Autodesk Inventor part; units mm, degrees
ref_plane "YZ Plane" through (0, 0, 0) normal (1, 0, 0) x (0, 1, 0)
ref_plane "XZ Plane" through (0, 0, 0) normal (0, 1, 0) x (-1, 0, 0)
ref_plane "XY Plane" through (0, 0, 0) normal (0, 0, 1) x (1, 0, 0)
sketch "スケッチ1" plane through (0, 0, 0) normal (0, 0, 1) x (1, 0, 0)
  line L0 (-23, 23) -> (23, 23)
  line L1 (23, 23) -> (23, -23)
  line L2 (23, -23) -> (-23, -23)
  line L3 (-23, -23) -> (-23, 23)
  point P0 (0, 0)
  dimension "d0" = 46
  dimension "d1" = 46
  dimension "d2" = 23
  dimension "d3" = 23
extrude "押し出し1" add sketch "スケッチ1" along normal blind 14.5
sketch "スケッチ2" plane through (23, -23, 0) normal (1, 0, 0) x (0, 0, -1)
  line L0 (0, 0) -> (-14.5, 0)
  line L1 (0, 46) -> (-14.5, 46)
  circle A0 centre (-12.25, 38) radius 1
  circle A1 centre (-12.25, 8) radius 1
  circle A2 centre (-12.25, 23) radius 1
  line L2 (-14.5, 46) -> (-14.5, 0)
  point P0 (0, 23)
  dimension "d6" = 2
  dimension "d8" = 8
  dimension "d13" = 8
  dimension "d14" = 15
  dimension "d48" = 2.25
  dimension "d49" = 2.25
  dimension "d50" = 2.25
hole "穴1" at (23, -15, 12.25) at (23, 0, 12.25) at (23, 15, 12.25) direction (-1, 0, 0) diameter 2 end through all
sketch "スケッチ3" plane through (-23, -23, 0) normal (0, -1, 0) x (1, 0, 0)
  line L0 (46, 14.5) -> (0, 14.5)
  line L1 (0, 0) -> (0, 14.5)
  line L2 (46, 0) -> (46, 14.5)
  circle A0 centre (8, 12.25) radius 1
  circle A1 centre (23, 12.25) radius 1
  circle A2 centre (38, 12.25) radius 1
  point P0 (23, 0)
  dimension "d22" = 2
  dimension "d23" = 2.25
  dimension "d24" = 2.25
  dimension "d25" = 2.25
  dimension "d26" = 8
  dimension "d27" = 8
  dimension "d28" = 15
hole "穴2" at (-15, -23, 12.25) at (15, -23, 12.25) at (0, -23, 12.25) direction (0, 1, 0) diameter 2 end through all
thread "ねじ1"
thread "ねじ2"
thread "ねじ3"
thread "ねじ4"
thread "ねじ5"
thread "ねじ6"
sketch "スケッチ4" plane through (0, 0, 14.5) normal (0, 0, 1) x (1, 0, 0)
  line L0 (-23, -23) -> (-23, 23)
  line L1 (23, -23) -> (-23, -23)
  circle A0 centre (-14, 19) radius 1.5
  circle A1 centre (8, 19) radius 1.5
  circle A2 centre (-14, -19) radius 1.5
  circle A3 centre (8, -19) radius 1.5
  dimension "d51" = 3
  dimension "d52" = 22
  dimension "d53" = 22
  dimension "d54" = 38
  dimension "d55" = 38
  dimension "d88" = 9
  dimension "d89" = 9
  dimension "d90" = 4
  dimension "d91" = 4
hole "穴3" at (-14, -19, 14.5) at (-14, 19, 14.5) at (8, -19, 14.5) at (8, 19, 14.5) direction (0, 0, -1) diameter 3 end through all
thread "ねじ7"
thread "ねじ8"
thread "ねじ9"
thread "ねじ10"
thread "ねじ11"
thread "ねじ12"
thread "ねじ13"
thread "ねじ14"
thread "ねじ15"
thread "ねじ16"
properties material "アセタール樹脂、白"
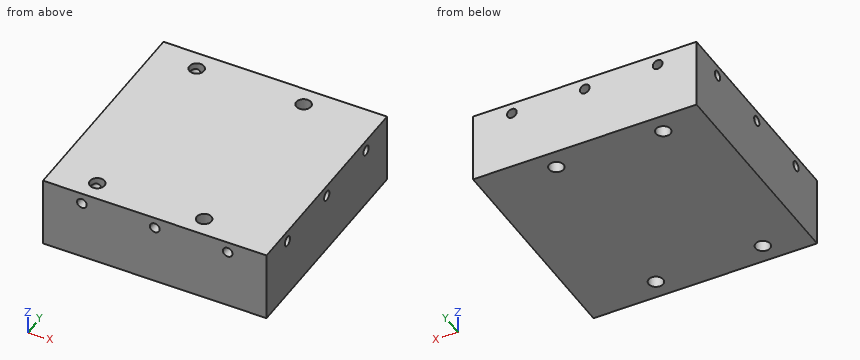
CAD build for the part. Positions are in the model's coordinates, mm. Round coordinates to 2 decimals unless told otherwise and drop trailing zeros. Write each loop counter-clockwise with the first axis right and the second up, starting at its lowest first coordinate (ties: lowest second). Pieces come first, ordered by that corner, then holes.
Item 1: Band-saw the part on C-C on z = 12.25. Give the number of separate pieces and of enclosed holes in the cut face, then the cut area to 3 significant figures.
Filled in:
separate pieces: 16
enclosed holes: 2
area: 1,580 mm2
Item 2: Drill centre lines: L1, parallel to Y at x = 17.5, z = 12.25; L2, parallel to X at y = -19, z = 5. Where is each one in solid material? Low to high.
Filled in:
L1: y = -23 to -16, -14 to -1, 1 to 14, 16 to 23
L2: x = -23 to -15.5, -12.5 to 6.5, 9.5 to 23
Item 3: Band-saw the part on B-B on y = -19. Write the cut outline in (x, z), then the cut area to 3 significant figures.
Filled in:
outline: (-23, 0) - (-15.5, 0) - (-15.5, 11.38) arc R1 cw to (-15.5, 13.12) - (-15.5, 14.5) - (-23, 14.5) - close; (-12.5, 0) - (6.5, 0) - (6.5, 14.5) - (-12.5, 14.5) - close; (9.5, 0) - (23, 0) - (23, 14.5) - (9.5, 14.5) - close; hole circle Ø2 at (0, 12.25); hole circle Ø2 at (15, 12.25)
area: 573 mm2
Item 4: Band-saw the part on A-A on x = 8. Write the cut outline in (y, z), then the cut area to 3 significant figures.
Filled in:
outline: (-23, 0) - (-20.5, 0) - (-20.5, 14.5) - (-23, 14.5) - close; (-17.5, 0) - (17.5, 0) - (17.5, 14.5) - (-17.5, 14.5) - close; (20.5, 0) - (23, 0) - (23, 14.5) - (20.5, 14.5) - close; hole circle Ø2 at (-15, 12.25); hole circle Ø2 at (0, 12.25); hole circle Ø2 at (15, 12.25)
area: 571 mm2
Item 5: Band-saw the part on D-D on y = 18.5. Write the cut outline in (x, z), then the cut area to 3 significant figures.
Filled in:
outline: (-23, 0) - (-15.41, 0) - (-15.41, 11.34) arc R1 cw to (-15.41, 13.16) - (-15.41, 14.5) - (-23, 14.5) - close; (-12.59, 0) - (6.59, 0) - (6.59, 14.5) - (-12.59, 14.5) - close; (9.41, 0) - (23, 0) - (23, 14.5) - (9.41, 14.5) - close; hole circle Ø2 at (0, 12.25); hole circle Ø2 at (15, 12.25)
area: 578 mm2
Item 6: Drop a flat-ended pin along its axis: pin 1 Ø1.6 at (x, z) = (0, 12.25) entering from -Y. Give the stop position or say it passes through.
Filled in:
pin 1: passes through
